```python
from build123d import *

# Parameters (mm, degrees)
SKETCH_6_R          = 20
EXTRUDE_6_DEPTH     = 20
SKETCH_8_W          = 30.6
SKETCH_8_H          = 2
CUT_EXTRUDE_2_DEPTH = 101
SKETCH_9_R          = 3.5
CUT_EXTRUDE_3_DEPTH = 77.97401861


with BuildPart() as part:
    # 草图6 → 凸台-拉伸6 (new body)
    with BuildSketch(Plane.XY.offset(-10)):
        with BuildLine():
            Line((-50, 0), (50, 0))
            Line((50, 0), (50, 32))
            Line((50, 32), (29.1719, 32))
            ThreePointArc((29.1719, 32), (0, 54.999995827), (-29.1719, 32))
            Line((-29.1719, 32), (-50, 32))
            Line((-50, 32), (-50, 0))
        make_face()
        with Locations((0, 25)):
            Circle(SKETCH_6_R, mode=Mode.SUBTRACT)
    extrude(amount=EXTRUDE_6_DEPTH)

    # 草图8 → 切除-拉伸2 (cut, symmetric)
    with BuildSketch(Plane.XY.offset(-10)):
        with Locations((35.7, 25)):
            Rectangle(SKETCH_8_W, SKETCH_8_H)
        with Locations((-35.7, 25)):
            Rectangle(SKETCH_8_W, SKETCH_8_H)
    extrude(amount=CUT_EXTRUDE_2_DEPTH, both=True, mode=Mode.SUBTRACT)

    # 草图9 → 切除-拉伸3 (cut, through all)
    with BuildSketch(Plane.XY.offset(-10)):
        with Locations((-40, 25)):
            Circle(SKETCH_9_R)
        with Locations((40, 25)):
            Circle(SKETCH_9_R)
    extrude(amount=CUT_EXTRUDE_3_DEPTH, mode=Mode.SUBTRACT)


solid = part.part
```
Geometry check sheet. Reference: the model listing, model coordinates, mm. A direction names the side the tool comes from. Give positions to 0.01 mm unless a question says otherwise; leave off trailing zeros. Order: outer loops, then holes, each group sorted by start corner. A loop starts at its lowest first (then second) coordinate and runs counter-clockwise, first axis right, second up. Notation, with made-up numbers: (-40, -17.5) - (-23, -17.5) arc R12 cw to (-23, -2.5) - close; hole circle Ø10 at (7, -34). An arc over 180 degrees is marked (long way). Answer in a Markdown table with one row per item. Add a question column.
Q1. Cross-section at C-C, the plane z = 2.25. Enter the section's corners in (x, y), then the cut area to 3 significant figures.
Q2. Material ranges on probe 1 along Y at (x, z) = (-35.5, 1.75); probe 2 along Y at (x, z) = (-0.5, 4.5); probe 3 along X at (y, z) = (34.5, -6), recorded low to high. Write a range as from..to.
Q3. Mould release check, pull along Y, two halves, no side actions. Record for faces 4 (the flat face through (40, 32, 0)), 5 (the flat face through (-1, 0, 0)), 6 (the flat face through (-20.4, 25, 0)): pulls with the +Y half, pulls with the -Y half, needs draft (parallel to the pull), parting line crosses it, or undercut.
Q4. Cross-section at D-D, the plane y = 49. Enter the section's corners in (x, z), then the cut area to 3 significant figures.
Q5. Cross-section at B-B, the plane x = 0. Enter the section's corners in (y, z), then the cut area to 3 significant figures.
Q6. Tool access check on faces 1 (the flat face through (-47, 26, 0)), 2 (the flat face through (20.4, 25, 0)), 3 (the cylindrical face through (-39.9, 28.5, -0.1)). Record the directions out of +Z, -Z, +X, -X, +Y, -Y that give a thin tool (end or side, any length) a straight path to the whole face; none if there is none.
Q7. Cross-section at A-A, the plane y = 25. Enter the section's corners in (x, z).
Q8. Gauge pin test, flat ends, axial feed: pin 1 (1 mm diameter, centred on y = 35, z = 2, fed in from -X); pin 2 (10 mm diameter, centred on x = 39, z = -4.5, fed in from +Y); pin 3 (1.6 mm diameter, centred on y = 25, z = -3.5, fed in from -X). Record the tip position at first contact, or that the pin passes through.
Check values:
| question | item | result |
|---|---|---|
| 1 | outline | (-50, 0) - (50, 0) - (50, 24) - (43.35, 24) arc R3.5 cw to (36.65, 24) - (20.4, 24) - (20.4, 26) - (36.65, 26) arc R3.5 cw to (43.35, 26) - (50, 26) - (50, 32) - (29.17, 32) arc R30 ccw to (-29.17, 32) - (-50, 32) - (-50, 26) - (-43.35, 26) arc R3.5 cw to (-36.65, 26) - (-20.4, 26) - (-20.4, 24) - (-36.65, 24) arc R3.5 cw to (-43.35, 24) - (-50, 24) - close; hole circle Ø40 at (0, 25) |
| 1 | area | 2,770 mm^2 |
| 2 | probe 1 | y = 0..24, 26..32 |
| 2 | probe 2 | y = 0..5.01, 44.99..55 |
| 2 | probe 3 | x = -28.46..-17.6, 17.6..28.46 |
| 3 | face 4 | pulls with the +Y half |
| 3 | face 5 | pulls with the -Y half |
| 3 | face 6 | undercut |
| 4 | outline | (-18, -10) - (18, -10) - (18, 10) - (-18, 10) - close |
| 4 | area | 720 mm^2 |
| 5 | outline | (0, -10) - (5, -10) - (5, 10) - (0, 10) - close; (45, -10) - (55, -10) - (55, 10) - (45, 10) - close |
| 5 | area | 300 mm^2 |
| 6 | face 1 | +Z, -Z, -X |
| 6 | face 2 | +Z, -Z, +X |
| 6 | face 3 | +Z, -Z |
| 7 | outline | (-20.4, -10) - (-20, -10) - (-20, 10) - (-20.4, 10) - close; (20, -10) - (20.4, -10) - (20.4, 10) - (20, 10) - close |
| 8 | pin 1 | stops at x = -28.46 |
| 8 | pin 2 | stops at y = 32 |
| 8 | pin 3 | stops at x = -20.4 |
